from build123d import *

# Parameters (mm, degrees)
CYLINDER002_R     = 3.14
CYLINDER002_DEPTH = 8
CYLINDER003_R     = 2.05
CYLINDER003_DEPTH = 14
BOX002_W          = 3.1
BOX002_H          = 0.39
BOX002_DEPTH      = 8.2


with BuildPart() as part:
    # Cylinder002 → Cylinder002 (join)
    with BuildSketch(Plane.XY.offset(4)):
        Circle(CYLINDER002_R)
    extrude(amount=CYLINDER002_DEPTH)

    # Cylinder003 → Cylinder003 (cut)
    with BuildSketch(Plane.XY.offset(3)):
        Circle(CYLINDER003_R)
    extrude(amount=CYLINDER003_DEPTH, mode=Mode.SUBTRACT)

    # Box002 → Box002 (cut)
    with BuildSketch(Plane(origin=(-1.55, 1.72, 3.9), x_dir=(1, 0, 0), z_dir=(0, 0, 1))):
        with Locations((1.55, 0.195)):
            Rectangle(BOX002_W, BOX002_H)
    extrude(amount=BOX002_DEPTH, mode=Mode.SUBTRACT)


solid = part.part
Geometry check sheet. Reference: the model listing, model coordinates, mm. Round coordinates to 2 decimals unless told otherwise and drop trailing zeros. Write each loop counter-clockwise with the first axis right and the second up, starting at its lowest first coordinate (ties: lowest second). Pieces come first, ordered by that corner, then holes.
Item 1: Section check A-A (x = 0). Record the boundary of the cut face in (y, z), plus the area to 3 significant figures.
Determined:
outline: (-3.14, 4) - (-2.05, 4) - (-2.05, 12) - (-3.14, 12) - close; (2.11, 4) - (3.14, 4) - (3.14, 12) - (2.11, 12) - close
area: 17.0 mm2
Item 2: Material ranges on line 1 along Y through (x, z) = (0, 6.5); line 2 along Y through (x, z) = (-1.5, 9); line 3 along Y through (x, z) = (0.75, 4.75), recorded low to high.
Determined:
line 1: y = -3.14 to -2.05, 2.11 to 3.14
line 2: y = -2.76 to -1.4, 1.4 to 1.72, 2.11 to 2.76
line 3: y = -3.05 to -1.91, 2.11 to 3.05
Item 3: Section check B-B (y = 0). Record the boundary of the cut face in (x, z), plus the area to 3 significant figures.
Determined:
outline: (-3.14, 4) - (-2.05, 4) - (-2.05, 12) - (-3.14, 12) - close; (2.05, 4) - (3.14, 4) - (3.14, 12) - (2.05, 12) - close
area: 17.4 mm2
Item 4: Mould release check, pull along X, two halves, no side actions. Record for faces 1 (the face through (2, -1, 4)), 2 (the face through (0, 2.11, 8)), 3 (the face through (2.995, 0.943, 7.944)): +X half, -X half, draft (parallel to the pull), parting line (faces both ways), or undercut.
Determined:
face 1: draft
face 2: undercut
face 3: parting line
Item 5: Section check D-D (x = -2.25). Record the boundary of the cut face in (y, z), plus the area to 3 significant figures.
Determined:
outline: (-2.19, 4) - (2.19, 4) - (2.19, 12) - (-2.19, 12) - close
area: 35.0 mm2
Item 6: Go/stop test with flat-tipped pins: pin 1 Ø0.5 at (x, z) = (1.5, 6.5) entering from +Y; pin 2 Ø3 at (y, z) = (2, 5) entering from +X; pin 3 Ø1 at (x, z) = (1.5, 6.5) entering from +Y. Record where each tip stops, or that it passes through.
Determined:
pin 1: stops at y = 2.88
pin 2: stops at x = 3.1
pin 3: stops at y = 2.98
Item 7: Section check C-C (z = 9.75). Record the boundary of the cut face in (x, y).
Determined:
outline: circle Ø6.28 at (0, 0); hole (-1.55, 1.72) - (-1.12, 1.72) arc R2.05 ccw (long way) to (1.12, 1.72) - (1.55, 1.72) - (1.55, 2.11) - (-1.55, 2.11) - close
